from build123d import *

# Parameters (mm, degrees)
SKETCH1_R                   = 2.3114
BOSS_EXTRUDE1_DEPTH         = 4.7625
F_14_0_182_DIAMETER_HOLE1_D = 4.6228
WEIGHTCUTTING_2_DEPTH       = 189.859131117
WEIGHTCUTTING_2_DEPTH_BACK  = 189.859131117
CUT_EXTRUDE1_DEPTH          = 189.859131117


with BuildPart() as part:
    # Sketch1 → Boss-Extrude1 (new body)
    with BuildSketch(Plane.XY):
        with BuildLine():
            Line((-168.768694788, 0), (168.768694788, 0))
            ThreePointArc((168.768694788, 0), (177.8, 31.75), (168.768694788, 63.5))
            Line((168.768694788, 63.5), (-168.768694788, 63.5))
            ThreePointArc((-168.768694788, 63.5), (-177.8, 31.75), (-168.768694788, 0))
        make_face()
        with Locations(Location((-117.475, 31.75, 0), (0, 0, 180))):
            Circle(SKETCH1_R, mode=Mode.SUBTRACT)
        with Locations(Location((117.475, 31.75, 0), (0, 0, 180))):
            Circle(SKETCH1_R, mode=Mode.SUBTRACT)
        with Locations(Location((-130.175, 31.75, 0), (0, 0, 180))):
            Circle(SKETCH1_R, mode=Mode.SUBTRACT)
        with Locations(Location((-104.775, 31.75, 0), (0, 0, 180))):
            Circle(SKETCH1_R, mode=Mode.SUBTRACT)
        with Locations(Location((104.775, 31.75, 0), (0, 0, 180))):
            Circle(SKETCH1_R, mode=Mode.SUBTRACT)
        with Locations(Location((130.175, 31.75, 0), (0, 0, 180))):
            Circle(SKETCH1_R, mode=Mode.SUBTRACT)
        with Locations(Location((-165.1, 57.15, 0), (0, 0, 180))):
            Circle(SKETCH1_R, mode=Mode.SUBTRACT)
        with Locations(Location((-165.1, 6.35, 0), (0, 0, 180))):
            Circle(SKETCH1_R, mode=Mode.SUBTRACT)
        with Locations(Location((165.1, 6.35, 0), (0, 0, 180))):
            Circle(SKETCH1_R, mode=Mode.SUBTRACT)
        with Locations(Location((165.1, 57.15, 0), (0, 0, 180))):
            Circle(SKETCH1_R, mode=Mode.SUBTRACT)
    extrude(amount=BOSS_EXTRUDE1_DEPTH)

    # #14 (0.182) Diameter Hole1 (through all)
    with Locations(Plane.XY.offset(4.7625)):
        with Locations((-73.088746639, 54.770291494), (-73.088746639, 42.070291494), (-73.088746639, 29.370291494), (-34.988746639, 29.370291494), (-34.988746639, 42.070291494), (-34.988746639, 54.770291494), (34.988746639, 54.770291494), (34.988746639, 42.070291494), (34.988746639, 29.370291494), (73.088746639, 29.370291494), (73.088746639, 42.070291494), (73.088746639, 54.770291494), (0, 44.45), (0, 31.75), (0, 19.05), (-6.35, 6.35), (6.35, 6.35)):
            Hole(F_14_0_182_DIAMETER_HOLE1_D / 2)

    # Sketch7 → WeightCutting_2 (cut, two sides: drawn at the far end of the back side and taken through both)
    with BuildSketch(Plane.XY.offset(4.7625).offset(-WEIGHTCUTTING_2_DEPTH_BACK)):
        with BuildLine():
            Line((-153.521805348, 54.441722315), (-137.644750023, 38.564666989))
            ThreePointArc((-137.644750023, 38.564666989), (-137.130061354, 38.220763016), (-136.522944675, 38.1))
            Line((-136.522944675, 38.1), (-81.818455145, 38.1))
            ThreePointArc((-81.818455145, 38.1), (-80.135747123, 38.797000484), (-79.438746639, 40.479708506))
            Line((-79.438746639, 40.479708506), (-79.438746639, 54.770291494))
            ThreePointArc((-79.438746639, 54.770291494), (-80.135747123, 56.452999516), (-81.818455145, 57.15))
            Line((-81.818455145, 57.15), (-152.4, 57.15))
            ThreePointArc((-152.4, 57.15), (-153.865709321, 56.170644342), (-153.521805348, 54.441722315))
        make_face()
        with BuildLine():
            Line((81.818455145, 57.15), (152.4, 57.15))
            ThreePointArc((152.4, 57.15), (153.865709321, 56.170644342), (153.521805348, 54.441722315))
            Line((153.521805348, 54.441722315), (137.644750023, 38.564666989))
            ThreePointArc((137.644750023, 38.564666989), (137.130061354, 38.220763016), (136.522944675, 38.1))
            Line((136.522944675, 38.1), (81.818455145, 38.1))
            ThreePointArc((81.818455145, 38.1), (80.135747123, 38.797000484), (79.438746639, 40.479708506))
            Line((79.438746639, 40.479708506), (79.438746639, 54.770291494))
            ThreePointArc((79.438746639, 54.770291494), (80.135747123, 56.452999516), (81.818455145, 57.15))
        make_face()
        with BuildLine():
            Line((-81.818455145, 6.35), (-152.4, 6.35))
            ThreePointArc((-152.4, 6.35), (-153.865709321, 7.329355658), (-153.521805348, 9.058277685))
            Line((-153.521805348, 9.058277685), (-137.644750023, 24.935333011))
            ThreePointArc((-137.644750023, 24.935333011), (-137.130061354, 25.279236984), (-136.522944675, 25.4))
            Line((-136.522944675, 25.4), (-81.818455145, 25.4))
            ThreePointArc((-81.818455145, 25.4), (-80.135747123, 24.702999516), (-79.438746639, 23.020291494))
            Line((-79.438746639, 23.020291494), (-79.438746639, 8.729708506))
            ThreePointArc((-79.438746639, 8.729708506), (-80.135747123, 7.047000484), (-81.818455145, 6.35))
        make_face()
        with BuildLine():
            Line((79.438746639, 23.020291494), (79.438746639, 8.729708506))
            ThreePointArc((79.438746639, 8.729708506), (80.135747123, 7.047000484), (81.818455145, 6.35))
            Line((81.818455145, 6.35), (152.4, 6.35))
            ThreePointArc((152.4, 6.35), (153.865709321, 7.329355658), (153.521805348, 9.058277685))
            Line((153.521805348, 9.058277685), (137.644750023, 24.935333011))
            ThreePointArc((137.644750023, 24.935333011), (137.130061354, 25.279236984), (136.522944675, 25.4))
            Line((136.522944675, 25.4), (81.818455145, 25.4))
            ThreePointArc((81.818455145, 25.4), (80.135747123, 24.702999516), (79.438746639, 23.020291494))
        make_face()
    extrude(amount=WEIGHTCUTTING_2_DEPTH + WEIGHTCUTTING_2_DEPTH_BACK, mode=Mode.SUBTRACT)

    # Sketch9 → Cut-Extrude1 (cut, through all)
    with BuildSketch(Plane.XY.offset(4.7625)):
        with BuildLine():
            Line((-47.688746639, 50.8), (-47.688746639, 12.7))
            ThreePointArc((-47.688746639, 12.7), (-54.038746639, 6.35), (-60.388746639, 12.7))
            Line((-60.388746639, 12.7), (-60.388746639, 50.8))
            ThreePointArc((-60.388746639, 50.8), (-54.038746639, 57.15), (-47.688746639, 50.8))
        make_face()
        with BuildLine():
            Line((60.388746639, 50.8), (60.388746639, 12.7))
            ThreePointArc((60.388746639, 12.7), (54.038746639, 6.35), (47.688746639, 12.7))
            Line((47.688746639, 12.7), (47.688746639, 50.8))
            ThreePointArc((47.688746639, 50.8), (54.038746639, 57.15), (60.388746639, 50.8))
        make_face()
        with BuildLine():
            Line((23.84437332, 50.8), (23.84437332, 12.7))
            ThreePointArc((23.84437332, 12.7), (17.49437332, 6.35), (11.14437332, 12.7))
            Line((11.14437332, 12.7), (11.14437332, 50.8))
            ThreePointArc((11.14437332, 50.8), (17.49437332, 57.15), (23.84437332, 50.8))
        make_face()
        with BuildLine():
            Line((-11.14437332, 50.8), (-11.14437332, 12.7))
            ThreePointArc((-11.14437332, 12.7), (-17.49437332, 6.35), (-23.84437332, 12.7))
            Line((-23.84437332, 12.7), (-23.84437332, 50.8))
            ThreePointArc((-23.84437332, 50.8), (-17.49437332, 57.15), (-11.14437332, 50.8))
        make_face()
    extrude(amount=-CUT_EXTRUDE1_DEPTH, mode=Mode.SUBTRACT)


solid = part.part
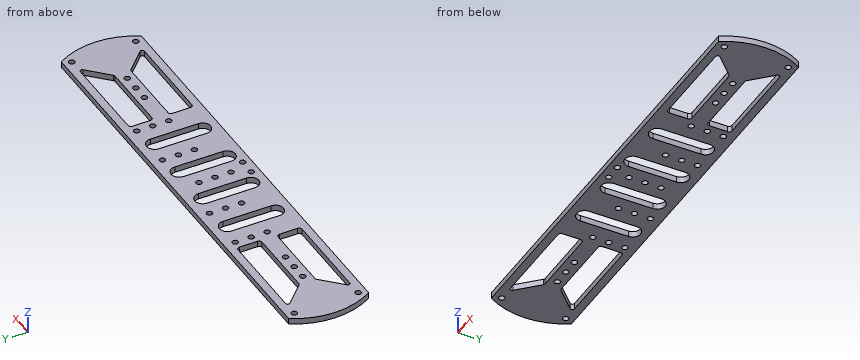
For this review, take the finished solid that the model builds, in its own axes (mm). Round coordinates to 2 decimals unless told otherwise and drop trailing zeros. Write each loop counter-clockwise with the first axis right and the second up, starting at its lowest first coordinate (ties: lowest second). Pieces come first, ordered by that corner, then holes. Notation, with made-up numbers: (19.25, 43) -> (49.25, 43) arc R20 ccw to (49.25, 54) -> close; hole circle Ø7 at (1, -26.5). An arc over 180 degrees is marked (long way). Use CSV: the item, a comma, the result in double quotes.
(1) Consider section A-A, the plane x = -87. Give the boundary of the cut face in (y, z), plus the area to 3 significant figures.
Computed values:
outline,"(0, 0) -> (6.35, 0) -> (6.35, 4.76) -> (0, 4.76) -> close; (25.4, 0) -> (38.1, 0) -> (38.1, 4.76) -> (25.4, 4.76) -> close; (57.15, 0) -> (63.5, 0) -> (63.5, 4.76) -> (57.15, 4.76) -> close"
area,"121 mm²"
(2) Consider section B-B, the plane z = 3.55. Give the number of separate pieces and of enclosed holes in the cut face, plus the area to 3 significant figures.
Computed values:
separate pieces,"1"
enclosed holes,"35"
area,"14,200 mm²"
(3) Clearance check with flat-ended pins moving along their axes: P1, Ø5.5, axis at x = 34.99, y = 54.77, coming from the -Z side; P2, Ø1.4, axis at y = 35, z = 1, coming from the -X side; P3, Ø1.5, axis at y = 10, z = 1.5, coming from the +X side; P4, Ø1.5, axis at y = 45, z = 3.5, coming from the -X side. State where each tip first meets the part, or that it passes through.
Computed values:
P1,"z = 0"
P2,"x = -177.75"
P3,"x = 174.03"
P4,"x = -176.49"
(4) To check wall thickness, follow L1, parallel to Y at x = 73, z = 0.9; L2, parallel to Y at x = -84, z = 2.45. State the ranges of each line that lie inside material, in increasing order. Write a range as [from, to].
Computed values:
L1,"[0, 27.06], [31.68, 39.76], [44.38, 52.46], [57.08, 63.5]"
L2,"[0, 6.35], [25.4, 38.1], [57.15, 63.5]"
